```python
from build123d import *

# Parameters (mm, degrees)
SKETCH1_W           = 628.65
SKETCH1_H           = 136.525
BOSS_EXTRUDE1_DEPTH = 12.7
CUT_EXTRUDE1_DEPTH  = 322.902569936
FILLET1_R           = 6.35


with BuildPart() as part:
    # Sketch1 → Boss-Extrude1 (new body)
    with BuildSketch(Plane(origin=(0, 0, 0), x_dir=(1, 0, 0), z_dir=(0, 1, 0))):
        Rectangle(SKETCH1_W, SKETCH1_H)
    extrude(amount=-BOSS_EXTRUDE1_DEPTH)

    # Sketch2 → Cut-Extrude1 (cut, through all)
    with BuildSketch(Plane(origin=(0, 0, 0), x_dir=(1, 0, 0), z_dir=(0, 1, 0))):
        Polygon((-250.825, -68.2625), (-244.475, -46.6725), (-155.575, -46.6725), (-149.225, -68.2625), align=None)
    extrude(amount=-CUT_EXTRUDE1_DEPTH, mode=Mode.SUBTRACT)

    # Fillet1
    fillet1_edges = [part.edges().sort_by_distance(p)[0] for p in [
        (-149.225, -6.35, 68.2625),
        (-250.825, -6.35, 68.2625),
        (-244.475, -6.35, 46.6725),
        (-155.575, -6.35, 46.6725),
    ]]
    fillet(fillet1_edges, radius=FILLET1_R)


solid = part.part
```
Geometry check sheet. Reference: the model listing, model coordinates, mm. A direction names the side the tool comes from. Coordinates: 2 decimals unless noted, no trailing zeros. Loops run counter-clockwise (first coordinate to the right, second up) from the corner with the lowest first, then second, coordinate; pieces in that order, holes last. Notation, with made-up numbers: (71, 19) - (116, 19) arc R14 cw to (116, 41) - close; hole circle Ø9 at (28, 43.5). An arc over 180 degrees is marked (long way). One line per item, written item: value. Start each with the question number.
(1) Depth check by flat-ended pin: P1, Ø3, axis at x = -198, y = -3.5, coming from the +Z side. Enter the tip coordinate at first touch or a pass-through.
(2) Cross-section at B-B on x = -208. Enter the section's corners in (y, z).
(3) Material ranges on line 1 (Z direction, x = -205, y = -9.75); line 2 (Z direction, x = -157, y = -3.75); line 3 (X direction, y = -8.5, z = 57.5) (3 decimals), recorded low to high. Write a range as [from, to].
(4) Tool access check on faces 4 (the flat face through (-247.676, -6.261, 57.555)), 5 (the flat face through (-4, -12.7, -1)). Record the directions out of +Z, -Z, +X, -X, +Y, -Y that give a thin tool (end or side, any length) a straight path to the whole face; none if there is none.
(5) Mould release check, pull along X, two halves, no side actions. Record for faces 1 (the flat face through (-4, 0, -1)), 2 (the flat face through (-201, -6, 46.672)), 3 (the flat face through (314.325, -6, 1)): released by +X, released by -X, zero draft, split by the parting line, or undercut.
Results below:
1. P1: stops at z = 46.67
2. outline: (-12.7, -68.26) - (0, -68.26) - (0, 46.67) - (-12.7, 46.67) - close
3. line 1: z = [-68.26, 46.67]
3. line 2: z = [-68.26, 47.61]
3. line 3: x = [-314.325, -247.66], [-152.39, 314.325]
4. face 4: +Z, +Y, -Y
4. face 5: +Z, -Z, +X, -X, -Y
5. face 1: zero draft
5. face 2: undercut
5. face 3: released by +X
